Geometry check sheet. Reference: the model listing, model coordinates, mm. A direction names the side the tool comes from. Give positions to 0.01 mm unless a question says otherwise; leave off trailing zeros. Order: outer loops, then holes, each group sorted by start corner. A loop starts at its lowest first (then second) coordinate and runs counter-clockwise, first axis right, second up. Notation, with made-up numbers: M 86,3.25 L 126,3.25 A23 ccw 126,38.25 Z; hole C 9.5,1 d11. An arc over 180 degrees is marked long. Answer as CSV lines item,"result".
from build123d import *

# Parameters (mm, degrees)
BASE_FLANGE1_DEPTH         = 75
SHEET_START                = -1
SHEET_METAL_STAMP1_DEPTH   = 1
SHEET_START_2              = -3
SHEET_METAL_STAMP1_2_DEPTH = 1
SHEET_START_3              = -2
SHEET_METAL_STAMP1_3_DEPTH = 1


# Read off the part's stored shape, not the designer's step: Sheet Metal Stamp1
# Sheet-metal steps are written as plain solids
with BuildPart() as part:
    # Sketch1 → Base-Flange1 (new, symmetric)
    with BuildSketch(Plane.YZ):
        with BuildLine():
            Line((50, 36), (39.420641265, 36))
            ThreePointArc((39.420641265, 36), (38.486121949, 35.768240269), (37.768186579, 35.126673649))
            Line((37.768186579, 35.126673649), (37.297724892, 34.436663175))
            ThreePointArc((37.297724892, 34.436663175), (36.938757207, 34.115879865), (36.471497549, 34))
            Line((36.471497549, 34), (34.057004901, 34))
            ThreePointArc((34.057004901, 34), (33.122485586, 33.768240269), (32.404550215, 33.126673649))
            Line((32.404550215, 33.126673649), (25.797724892, 23.436663175))
            ThreePointArc((25.797724892, 23.436663175), (25.438757207, 23.115879865), (24.971497549, 23))
            Line((24.971497549, 23), (24.499216659, 23))
            ThreePointArc((24.499216659, 23), (23.424617442, 22.686782892), (22.686601085, 21.845236523))
            Line((22.686601085, 21.845236523), (12.769237526, 0.577381738))
            ThreePointArc((12.769237526, 0.577381738), (12.400229348, 0.156608554), (11.862929739, 0))
            Line((11.862929739, 0), (-11.862929739, 0))
            ThreePointArc((-11.862929739, 0), (-12.400229348, 0.156608554), (-12.769237526, 0.577381738))
            Line((-12.769237526, 0.577381738), (-22.686601085, 21.845236523))
            ThreePointArc((-22.686601085, 21.845236523), (-23.424617442, 22.686782892), (-24.499216659, 23))
            Line((-24.499216659, 23), (-24.971497549, 23))
            ThreePointArc((-24.971497549, 23), (-25.438757207, 23.115879865), (-25.797724892, 23.436663175))
            Line((-25.797724892, 23.436663175), (-32.404550215, 33.126673649))
            ThreePointArc((-32.404550215, 33.126673649), (-33.122485586, 33.768240269), (-34.057004901, 34))
            Line((-34.057004901, 34), (-36.471497549, 34))
            ThreePointArc((-36.471497549, 34), (-36.938757207, 34.115879865), (-37.297724892, 34.436663175))
            Line((-37.297724892, 34.436663175), (-37.768186579, 35.126673649))
            ThreePointArc((-37.768186579, 35.126673649), (-38.486121949, 35.768240269), (-39.420641265, 36))
            Line((-39.420641265, 36), (-50, 36))
            Line((-50, 36), (-50, 35))
            Line((-50, 35), (-39.420641265, 35))
            ThreePointArc((-39.420641265, 35), (-38.953381607, 34.884120135), (-38.594413922, 34.563336825))
            Line((-38.594413922, 34.563336825), (-38.123952235, 33.873326351))
            ThreePointArc((-38.123952235, 33.873326351), (-37.406016865, 33.231759731), (-36.471497549, 33))
            Line((-36.471497549, 33), (-34.057004901, 33))
            ThreePointArc((-34.057004901, 33), (-33.589745243, 32.884120135), (-33.230777558, 32.563336825))
            Line((-33.230777558, 32.563336825), (-26.623952235, 22.873326351))
            ThreePointArc((-26.623952235, 22.873326351), (-25.906016865, 22.231759731), (-24.971497549, 22))
            Line((-24.971497549, 22), (-24.499216659, 22))
            ThreePointArc((-24.499216659, 22), (-23.961917051, 21.843391446), (-23.592908872, 21.422618262))
            Line((-23.592908872, 21.422618262), (-13.675545313, 0.154763477))
            ThreePointArc((-13.675545313, 0.154763477), (-12.937528956, -0.686782892), (-11.862929739, -1))
            Line((-11.862929739, -1), (11.862929739, -1))
            ThreePointArc((11.862929739, -1), (12.937528956, -0.686782892), (13.675545313, 0.154763477))
            Line((13.675545313, 0.154763477), (23.592908872, 21.422618262))
            ThreePointArc((23.592908872, 21.422618262), (23.961917051, 21.843391446), (24.499216659, 22))
            Line((24.499216659, 22), (24.971497549, 22))
            ThreePointArc((24.971497549, 22), (25.906016865, 22.231759731), (26.623952235, 22.873326351))
            Line((26.623952235, 22.873326351), (33.230777558, 32.563336825))
            ThreePointArc((33.230777558, 32.563336825), (33.589745243, 32.884120135), (34.057004901, 33))
            Line((34.057004901, 33), (36.471497549, 33))
            ThreePointArc((36.471497549, 33), (37.406016865, 33.231759731), (38.123952235, 33.873326351))
            Line((38.123952235, 33.873326351), (38.594413922, 34.563336825))
            ThreePointArc((38.594413922, 34.563336825), (38.953381607, 34.884120135), (39.420641265, 35))
            Line((39.420641265, 35), (50, 35))
            Line((50, 35), (50, 36))
        make_face()
    extrude(amount=BASE_FLANGE1_DEPTH, both=True)

    # Sheet Metal Stamp1 outline → Sheet Metal Stamp1 (cut)
    with BuildSketch(Plane.XY.offset(SHEET_START)):
        with BuildLine():
            ThreePointArc((-15, 9), (-24, 0), (-15, -9))
            Line((-15, -9), (15, -9))
            ThreePointArc((15, -9), (24, 0), (15, 9))
            Line((15, 9), (-15, 9))
        make_face()
    extrude(amount=SHEET_METAL_STAMP1_DEPTH, mode=Mode.SUBTRACT)



with BuildPart() as body_2:
    # Sheet Metal Stamp1 2 outline → Sheet Metal Stamp1 2 (new body)
    with BuildSketch(Plane.XY.offset(SHEET_START_2)):
        with BuildLine():
            ThreePointArc((-15, 10), (-25, 0), (-15, -10))
            Line((-15, -10), (15, -10))
            ThreePointArc((15, -10), (25, 0), (15, 10))
            Line((15, 10), (-15, 10))
        make_face()
    extrude(amount=SHEET_METAL_STAMP1_2_DEPTH)


with BuildPart() as part_1:
    add(part.part)

    add(body_2.part)  # Sheet Metal Stamp1 3 merges body 2
    # Sheet Metal Stamp1 3 outline → Sheet Metal Stamp1 3 (add)
    with BuildSketch(Plane.XY.offset(SHEET_START_3)):
        with BuildLine():
            ThreePointArc((-15, 10), (-25, 0), (-15, -10))
            Line((-15, -10), (15, -10))
            ThreePointArc((15, -10), (25, 0), (15, 10))
            Line((15, 10), (-15, 10))
        make_face()
        with BuildLine():
            Line((15, -9), (-15, -9))
            ThreePointArc((-15, -9), (-24, 0), (-15, 9))
            Line((-15, 9), (15, 9))
            ThreePointArc((15, 9), (24, 0), (15, -9))
        make_face(mode=Mode.SUBTRACT)
    extrude(amount=SHEET_METAL_STAMP1_3_DEPTH)


solid = part_1.part
(1) Section check A-A on y = 0. Enter the section's corners in (x, z).
The answers:
outline,"M -75,-1 L -25,-1 L -25,-3 L 25,-3 L 25,-1 L 75,-1 L 75,0 L 24,0 L 24,-2 L -24,-2 L -24,0 L -75,0 Z"
(2) Section check C-C on z = 26.5. Enter the section's corners in (x, y).
The answers:
outline,"M -75,-29.1 L 75,-29.1 L 75,-27.89 L -75,-27.89 Z; M -75,27.89 L 75,27.89 L 75,29.1 L -75,29.1 Z"
(3) Draft check along X on faces 5 (the face through (1, -45, 36)), 6 (the face through (24, 0, -1)), 7 (the face through (75, 18, 11)). Enter one of: +X half, -X half, draft (parallel to the pull), parting line (faces both ways), or undercut.
The answers:
face 5,"draft"
face 6,"undercut"
face 7,"+X half"
(4) Section check D-D on y = 30. Enter the section's corners in (x, z), then the cut area to 3 significant figures.
The answers:
outline,"M -75,27.82 L 75,27.82 L 75,29.6 L -75,29.6 Z"
area,"266 mm2"
(5) Tool access check on faces 1 (the face through (1, 45, 35)), 2 (the face through (1.05, 17.797, 11.36)), 3 (the face through (1, -45, 35)), 4 (the face through (-25, 0, -2)). Record the directions out of +Z, -Z, +X, -X, +Y, -Y that give a thin tool (end or side, any length) a straight path to the whole face; none if there is none.
The answers:
face 1,"-Z, +X, -X, +Y"
face 2,"+Z, +X, -X"
face 3,"-Z, +X, -X, -Y"
face 4,"-Z, -X"
(6) Material ranges on line 1 (Z direction, x = -60, y = -11.5); line 2 (Y direction, x = 25, z = 19); line 3 (Y direction, x = -0.5, z = 31.5), recorded low to high.
The answers:
line 1,"z = -1 to 0"
line 2,"y = -22.46 to -21.36, 21.36 to 22.46"
line 3,"y = -32.51 to -31.3, 31.3 to 32.51"
(7) Section check B-B on z = 9. Enter the section's corners in (x, y), then the cut area to 3 significant figures.
The answers:
outline,"M -75,-17.8 L 75,-17.8 L 75,-16.7 L -75,-16.7 Z; M -75,16.7 L 75,16.7 L 75,17.8 L -75,17.8 Z"
area,"331 mm2"
(8) Gauge pin test, flat ends, axial feed: P1, Ø9, axis at x = 4, y = -1, coming from the +Z side; P2, Ø3, axis at x = -6, y = -46.5, coming from the -Z side; P3, Ø5, axis at x = 44.5, z = 27.5, coming from the +Y side. Record the tip position at first contact, or that the pin passes through.
The answers:
P1,"stops at z = -2"
P2,"stops at z = 35"
P3,"stops at y = 31.48"
